Design review of the part built by this model. Coordinates are the model's own, in mm. A direction names the side the tool comes from. Give positions to 0.01 mm unless a question says otherwise; leave off trailing zeros. Write each loop counter-clockwise with the first axis right and the second up, starting at its lowest first coordinate (ties: lowest second). Pieces come first, ordered by that corner, then holes. Notation, with made-up numbers: (8.25, -26) -> (56.25, -26) arc R14 cw to (56.25, 1) -> close; hole circle Ø1 at (57.5, 2.25). An arc over 180 degrees is marked (long way). Use CSV: the item, a comma, the result in double quotes.
Autodesk Inventor part; units mm, degrees
ref_plane "YZ Plane" through (0, 0, 0) normal (1, 0, 0) x (0, 1, 0)
ref_plane "XZ Plane" through (0, 0, 0) normal (0, 1, 0) x (-1, 0, 0)
ref_plane "XY Plane" through (0, 0, 0) normal (0, 0, 1) x (1, 0, 0)
sketch "Sketch1" plane through (0, 0, 0) normal (0, 1, 0) x (-1, 0, 0)
  line L0 (-1.8331, -3.175) -> (-3.6662, 0)
  line L1 (-3.6662, 0) -> (-1.8331, 3.175)
  line L2 (-1.8331, 3.175) -> (1.8331, 3.175)
  line L3 (1.8331, 3.175) -> (3.6662, 0)
  line L4 (3.6662, 0) -> (1.8331, -3.175)
  line L5 (1.8331, -3.175) -> (-1.8331, -3.175)
  point P0 (0, 0)
  point P1 (0, 0)
  dimension "d0" = 6.35
extrude "Body" add sketch "Sketch1" along normal blind 76.2
sketch "Sketch2" plane through (0, 76.2, 0) normal (0, 1, 0) x (1, 0, 0)
  circle A0 centre (0, 0) radius 2.0955
  dimension "d3" = 4.191
extrude "Hole 2" cut sketch "Sketch2" against normal blind 12.7
sketch "Sketch3" plane through (0, 0, 0) normal (0, -1, 0) x (1, 0, 0)
  circle A0 centre (0, 0) radius 2.0955
  dimension "d6" = 4.191
extrude "Hole 1" cut sketch "Sketch3" against normal blind 12.7
chamfer "Hole 2 Chamfer 1" distance 0.127 distance2 0.1244 1 edges at (-2.0955, 76.2, 0) measured on face at (0.0842, 76.2, 2.8101)
chamfer "Hole 1 Chamfer 1" distance 0.127 distance2 0.1244 1 edges at (-2.0955, 0, 0) measured on face at (-0.0842, 0, 2.8101)
sketch "Sketch4" plane through (0, 0, 0) normal (0, 0, 1) x (1, 0, 0)
  line L0 (1.8331, 76.2) -> (-1.8331, 76.2)
  line L1 (0, 76.2) -> (-3.0353, 76.2)
  line L2 (-3.6662, 76.2) -> (-1.8331, 76.2)
  line L3 (-3.6662, 0) -> (-3.6662, 76.2)
  arc A0 (-3.0353, 76.2) -> (-3.6662, 75.565) centre (-2.2234, 74.7624) ccw
  line L4 (-3.6662, 75.565) -> (-6.3588, 78.1647)
  line L5 (-6.3588, 78.1647) -> (0, 76.2)
  line L6 (0, 76.2) -> (0, 129.864)
  point P0 (0, 0)
  dimension "d15" = 3.0353
  dimension "d16" = 1.651
  dimension "d17" = 0.635
revolve "Hole 2 Chamfer 2" cut sketch "Sketch4" angle 360 about axis through (0, 76.2, 0) along (0, 1, 0)
sketch "Sketch5" plane through (0, 0, 0) normal (0, 0, 1) x (1, 0, 0)
  line L0 (0, 0) -> (-3.0353, 0)
  line L1 (1.8331, 0) -> (-1.8331, 0)
  line L2 (-3.6662, 0) -> (-3.6662, 76.2)
  arc A0 (-3.6662, 0.635) -> (-3.0353, 0) centre (-2.2234, 1.4376) ccw
  line L3 (0, 0) -> (0, -2.1986)
  line L4 (-3.6662, 0.635) -> (-4.1154, -0.8715)
  line L5 (-4.1154, -0.8715) -> (0, 0)
  point P0 (-3.6662, 75.565)
  dimension "d19" = 3.0353
  dimension "d20" = 1.651
  dimension "d21" = 0.635
revolve "Hole 1 Chamfer 2" cut sketch "Sketch5" angle 360 about axis through (0, 0, 0) along (0, -1, 0)
chamfer "Hole 2 Chamfer 1 For Short" [suppressed]
sketch "Sketch7" plane through (0, 0, 0) normal (0, 0, 1) x (1, 0, 0)
  line L0 (0, 76.2004) -> (3.0353, 76.2)
  line L1 (3.6662, 76.2) -> (1.8331, 76.2)
  line L2 (3.6662, 0.635) -> (3.6662, 76.2)
  arc A0 (3.6662, 75.565) -> (3.0353, 76.2) centre (2.2234, 74.7624) ccw
  line L3 (3.6662, 75.565) -> (4.2663, 77.1032)
  line L4 (4.2663, 77.1032) -> (0, 76.2004)
  line L5 (0, 78.0061) -> (0, 76.2004)
  line L6 (1.8331, 76.2) -> (-1.8331, 76.2)
  point P0 (0, 0)
  point P1 (0, 76.2)
  dimension "d33" = 3.0353
  dimension "d34" = 1.651
  dimension "d35" = 0.635
revolve "Hole 2 Chamfer 2 For Short" [suppressed]
properties part number "Standoff .5" material "VEX Aluminum Alloy 5052-H32"
(1) For line 1 along Z through (x, y) = (0, 68.25) (1 decimal); line 2 along X through (y, z) = (72.5, 0); line 3 along Y through (x, z) = (-2, -0.5), list the stretches that pass through material, from the lowest coordinate up. Write a range as [from, to].
Established:
line 1,"z = [-3.2, -2.1], [2.1, 3.2]"
line 2,"x = [-3.67, -2.1], [2.1, 3.67]"
line 3,"y = [12.7, 63.5]"
(2) Take a section at A-A (y = 64.5). Write out the cut boundary in (x, z) (1 decimal).
Established:
outline,"(-3.7, 0) -> (-1.8, -3.2) -> (1.8, -3.2) -> (3.7, 0) -> (1.8, 3.2) -> (-1.8, 3.2) -> close; hole circle Ø4.2 at (0, 0)"
(3) Tool access review of faces 1 (the face through (0, 38, -3.175)), 2 (the face through (0, 63.5, 0)), 3 (the face through (2, 6.32, 0.63)): name each direction out of +Z, -Z, +X, -X, +Y, -Y from which nothing blocks a thin tool from reaching the whole face with its end or side.
Established:
face 1,"-Z, +X, -X, +Y, -Y"
face 2,"+Y"
face 3,"-Y"
(4) Mouldability with a two-part tool opening along Z and no side actions: class faces 4 (the face through (2.76, 37.57, 1.57)), 5 (the face through (2, 76.2, 2)), 6 (the face through (0, 12.7, 0)) as +Z half, -Z half, draft (parallel to the pull), parting line (faces both ways), or undercut.
Established:
face 4,"+Z half"
face 5,"draft"
face 6,"undercut"
(5) Take a section at C-C (y = 48.5). Write out the cut boundary in (x, z) (3 decimals), then the cut area to 3 significant figures.
Established:
outline,"(-3.666, 0) -> (-1.833, -3.175) -> (1.833, -3.175) -> (3.666, 0) -> (1.833, 3.175) -> (-1.833, 3.175) -> close"
area,"34.9 mm2"
(6) Clearance check with flat-ended pins moving along their axes: pin 1 (3 mm diameter, centred on y = 49, z = 1, fed in from -X); pin 2 (2 mm diameter, centred on x = -0.5, z = -0.5, fed in from +Y). State where each tip first meets the part, or that it passes through.
Established:
pin 1,"stops at x = -3.67"
pin 2,"stops at y = 63.5"
